Here's the drawing with two shaded views (mm, measured from the low corner). I have some questions. A direction names the side the tool comes from. Give positions to 0.01 mm unless a question says otherwise; leave off trailing zeros. Loops run counter-clockwise (first coordinate to the right, second up) from the corner with the lowest first, then second, coordinate; pieces in that order, holes last.
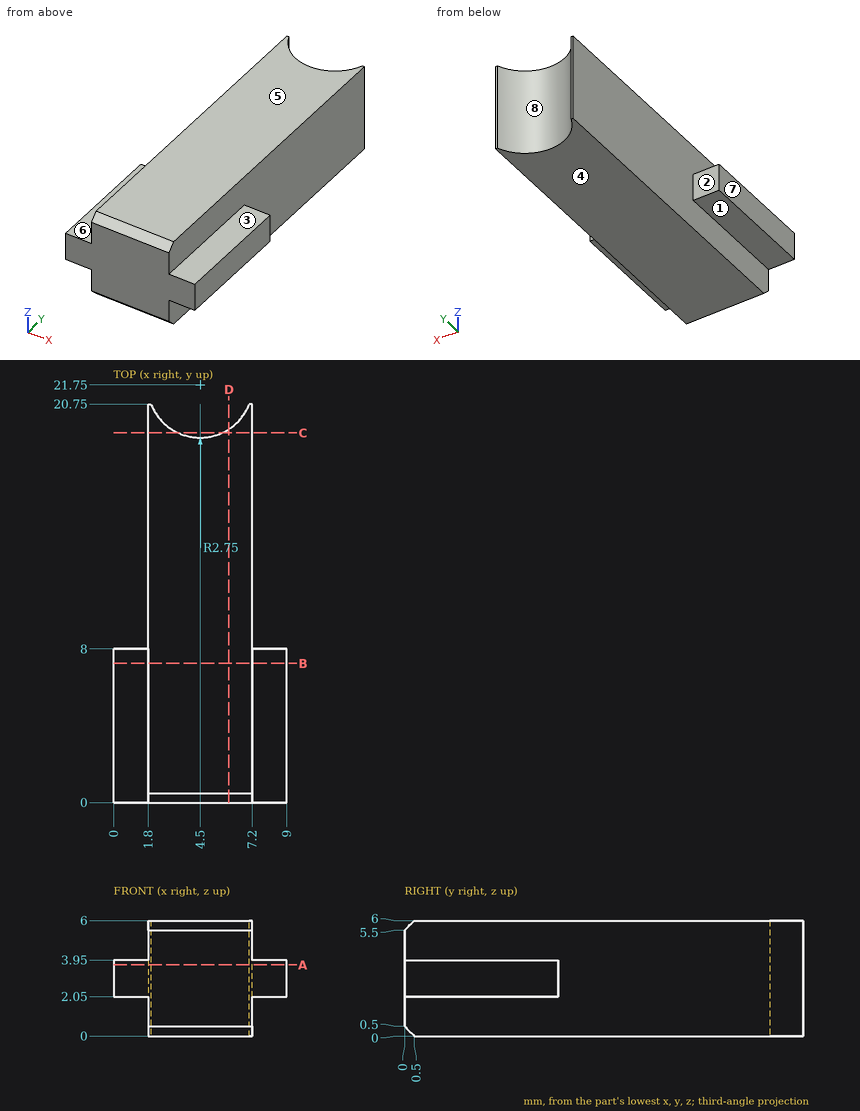
(1) Which directions (+Z, -Z, +X, -X, +Y, -Y) give clear straight access to the entire face, cutting with the end or side of a thin tool? Please do the marked faces 1, 2, 3, 4 and 5.
Returned:
face 1: -Z, -X, +Y, -Y
face 2: +Z, -Z, -X, +Y
face 3: +Z, +X, +Y, -Y
face 4: -Z, +X, -X, +Y, -Y
face 5: +Z, +X, -X, +Y, -Y
(2) Suppose I cut it at D-D on x = 6. List the corners of the cut face in (y, z) for me.
Returned:
outline: (0, 0.5) - (0.5, 0) - (19.45, 0) - (19.45, 6) - (0.5, 6) - (0, 5.5) - close
(3) Thinking about a two-plate mould opening in X: for the marked faces 6, 7 and 8, which applies, pulls with the +X half, pulls with the -X half, needs draft (parallel to the pull), parting line crosses it, or undercut?
Returned:
face 6: needs draft
face 7: pulls with the -X half
face 8: undercut
(4) Please list where these lines run through material, in increasing order: probe 1 along X at (y, z) = (14.5, 4.2); probe 2 along Z at (x, y) = (1, 5.25); probe 3 along Y at (x, z) = (4.5, 0.65).
Returned:
probe 1: x = 1.8 to 7.2
probe 2: z = 2.05 to 3.95
probe 3: y = 0 to 19
(5) Will these pins go through, and if not, where does the flat tip stop? P1, Ø3, axis at y = 14.5, z = 2, coming from the -X side; P2, Ø2, axis at x = 8.5, y = 3, coming from the -Z side; P3, Ø0.9, axis at x = 8, z = 3, coming from the +Y side.
Returned:
P1: stops at x = 1.8
P2: stops at z = 2.05
P3: stops at y = 8
(6) Suppose I cut it at A-A on z = 3.7. List the corners of the cut face in (x, y) for me, plus the area to 3 significant figures.
Returned:
outline: (0, 0) - (9, 0) - (9, 8) - (7.2, 8) - (7.2, 20.75) - (7.06, 20.75) arc R2.75 cw to (1.94, 20.75) - (1.8, 20.75) - (1.8, 8) - (0, 8) - close
area: 134 mm2
(7) Suppose I cut it at B-B on y = 7.25. List the corners of the cut face in (x, z) for me, plus the area to 3 significant figures.
Returned:
outline: (0, 2.05) - (1.8, 2.05) - (1.8, 0) - (7.2, 0) - (7.2, 2.05) - (9, 2.05) - (9, 3.95) - (7.2, 3.95) - (7.2, 6) - (1.8, 6) - (1.8, 3.95) - (0, 3.95) - close
area: 39.2 mm2
(8) Suppose I cut it at C-C on y = 19.25. List the corners of the cut face in (x, z) for me, plus the area to 3 significant figures.
Returned:
outline: (1.8, 0) - (3.35, 0) - (3.35, 6) - (1.8, 6) - close; (5.65, 0) - (7.2, 0) - (7.2, 6) - (5.65, 6) - close
area: 18.7 mm2
